```python
from build123d import *

# Parameters (mm, degrees)
F1_DEPTH = 19.05
F2_W     = 38.1
F2_H     = 38.1
F3_DEPTH = 19.05
F4_W     = 38.1
F4_H     = 38.1
F4_W_2   = 19.05
F4_H_2   = 19.05
F5_DEPTH = 19.05


with BuildPart() as f1:
    # F0 (on Top) → F1 (new body, symmetric)
    with BuildSketch(Plane.XY):
        Polygon((152.4, -19.05), (152.4, 19.05), (-114.3, 19.05), (-152.4, -19.05), align=None)
    extrude(amount=F1_DEPTH, both=True)

    # F2 (on Top) → F3 (cut)
    with BuildSketch(Plane.XY):
        Rectangle(F2_W, F2_H)
    extrude(amount=F3_DEPTH, mode=Mode.SUBTRACT)

    # F4 (on face) → F5 (cut)
    with BuildSketch(Plane.YZ.offset(152.4)):
        Rectangle(F4_W, F4_H)
        Rectangle(F4_W_2, F4_H_2, mode=Mode.SUBTRACT)
    extrude(amount=-F5_DEPTH, mode=Mode.SUBTRACT)


solid = f1.part
```
The listing builds one solid part. Answer for the finished solid, in the listing's coordinates (mm). A direction names the side the tool comes from. Give positions to 0.01 mm unless a question says otherwise; leave off trailing zeros. Order: outer loops, then holes, each group sorted by start corner. A loop starts at its lowest first (then second) coordinate and runs counter-clockwise, first axis right, second up. Notation, with made-up numbers: (-2.5, 58) -> (13.5, 58) arc R24 ccw to (13.5, 87) -> close; hole circle Ø11 at (58, 79.5). An arc over 180 degrees is marked (long way). One line per item, written item: value.
1) Find section D-D, the plane z = -15. Determine the outline of the cut face in (x, y).
Reported:
outline: (-152.4, -19.05) -> (133.35, -19.05) -> (133.35, 19.05) -> (-114.3, 19.05) -> close
2) Find the intervals of material crossed by line 1 (X direction, y = 8.5, z = 5); line 2 (X direction, y = -9, z = 16); line 3 (Z direction, x = 2.5, y = -11), in increasing order.
Reported:
line 1: x = -124.85 to -19.05, 19.05 to 152.4
line 2: x = -142.35 to -19.05, 19.05 to 133.35
line 3: z = -19.05 to 0
3) A tool of negligible diameter and unlimited length cuts with its end or side. For faces 1 (the flat face through (143, 0, -9.525)), 2 (the flat face through (-19.05, 0, 9)), 3 (the flat face through (143, 9.525, 0)), 4 (the flat face through (143, -9.525, 0)), 5 (the flat face through (-133.08, 0.27, 0.27)), from which of +Z, -Z, +X, -X, +Y, -Y can it reach the whole face along a straight path? Write none if from no direction.
Reported:
face 1: -Z, +X, +Y, -Y
face 2: +Z, +Y, -Y
face 3: +Z, -Z, +X, +Y
face 4: +Z, -Z, +X, -Y
face 5: +Z, -Z, -X, +Y
4) Determine the mould class of faces 6 (the flat face through (143, 0, 9.525)), 7 (the flat face through (152.4, 0, 0)), 8 (the flat face through (19.05, 0, 9)) for opening direction X: pulls with the +X half, pulls with the -X half, needs draft (parallel to the pull), parting line crosses it, or undercut.
Reported:
face 6: needs draft
face 7: pulls with the +X half
face 8: undercut
5) Find section A-A, the plane z = 2.5. Determine the outline of the cut face in (x, y) (3 decimals).
Reported:
outline: (-152.4, -19.05) -> (-19.05, -19.05) -> (-19.05, 19.05) -> (-114.3, 19.05) -> close; (19.05, -19.05) -> (133.35, -19.05) -> (133.35, -9.525) -> (152.4, -9.525) -> (152.4, 9.525) -> (133.35, 9.525) -> (133.35, 19.05) -> (19.05, 19.05) -> close
6) Find section C-C, the plane x = -131. Determine the outline of the cut face in (y, z), plus the area to 3 significant figures.
Reported:
outline: (-19.05, -19.05) -> (2.35, -19.05) -> (2.35, 19.05) -> (-19.05, 19.05) -> close
area: 815 mm^2
7) Find section B-B, the plane y = 5. Determine the outline of the cut face in (x, z) (3 decimals), plus the area to 3 significant figures.
Reported:
outline: (-128.35, -19.05) -> (133.35, -19.05) -> (133.35, -9.525) -> (152.4, -9.525) -> (152.4, 9.525) -> (133.35, 9.525) -> (133.35, 19.05) -> (19.05, 19.05) -> (19.05, 0) -> (-19.05, 0) -> (-19.05, 19.05) -> (-128.35, 19.05) -> close
area: 9,610 mm^2
8) Flat-ended cylindrical pins translate along their axes: P1, Ø21, axis at y = 1.5, z = 5.5, coming from the -X side; P2, Ø12, axis at y = -11, z = 12.5, coming from the -X side; P3, Ø9.5, axis at x = 141.5, z = -4.5, coming from the -Y side (3 decimals); P4, Ø3, axis at x = 9.5, z = 2.5, coming from the +Y side. Find the tip coordinate at first contact, or state that the pin passes through.
Reported:
P1: stops at x = -142.35
P2: stops at x = -150.35
P3: stops at y = -9.525
P4: passes through
